Verification items for the finished model (mm, model axes). Round coordinates to 2 decimals unless told otherwise and drop trailing zeros. Order: outer loops, then holes, each group sorted by start corner. A loop starts at its lowest first (then second) coordinate and runs counter-clockwise, first axis right, second up. Notation, with made-up numbers: (-25.5, -12) -> (17.5, -12) arc R22 cw to (17.5, 26) -> close; hole circle Ø11 at (18.25, 18). An arc over 180 degrees is marked (long way). Answer in a Markdown table with one row per item. Add a question column.
```python
from build123d import *

# Parameters (mm, degrees)
F0_R = 4.953


with BuildPart() as f2:
    # F2: sweep along a path in F1
    with BuildLine(Plane.YZ) as f2_path:
        Line((0, 0), (0, 152.4))
        Line((0, 152.4), (304.8, 152.4))
        Line((304.8, 152.4), (304.8, -609.6))
        Line((304.8, -609.6), (1371.6, -609.6))
        Line((1371.6, -609.6), (1371.6, -457.2))
    # F0 (on Top) → F2 (sweep)
    with BuildSketch(Plane.XY):
        Circle(F0_R)
    sweep(path=f2_path.line, transition=Transition.RIGHT)


solid = f2.part
```
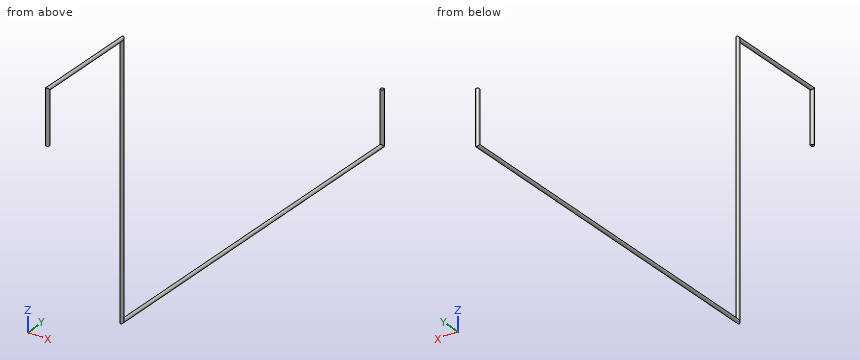
1) Depth check by flat-ended pin: P1, Ø1, axis at x = 1.5, z = -277.5, coming from the +Y side; P2, Ø2, axis at x = 2, y = 239, coming from the -Z side; P3, Ø3, axis at x = -2, y = 584, coming from the -Z side. Enter the tip coordinate at first touch or a pass-through.
2) Cross-section at D-D, the plane z = -320.5. Record the boundary of the cut face in (x, y).
3) Cross-section at A-A, the plane x = 0. Record the boundary of the cut face in (y, z).
4) Thickness scan on L1, parallel to Y at x = 1.25, z = 12.5; L2, parallel to Y at x = 0.5, z = -463; L3, parallel to Z at x = 1.5, y = 196. Record the ranges inside material, lowest first. Write a range as [from, to].
5) Cross-section at C-C, the plane y = 550.5. Record the boundary of the cut face in (x, z).
6) Cross-section at B-B, the plane z = 93. Record the boundary of the cut face in (x, y).
Results below:
| question | item | result |
|---|---|---|
| 1 | P1 | y = 309.65 |
| 1 | P2 | z = 147.55 |
| 1 | P3 | z = -614.53 |
| 2 | outline | circle Ø9.91 at (0, 304.8) |
| 3 | outline | (-4.95, 0) -> (4.95, 0) -> (4.95, 147.45) -> (299.85, 147.45) -> (299.85, -614.55) -> (1376.55, -614.55) -> (1376.55, -457.2) -> (1366.65, -457.2) -> (1366.65, -604.65) -> (309.75, -604.65) -> (309.75, 157.35) -> (-4.95, 157.35) -> close |
| 4 | L1 | [-4.79, 4.79], [300.01, 309.59] |
| 4 | L2 | [299.87, 309.73], [1366.67, 1376.53] |
| 4 | L3 | [147.68, 157.12] |
| 5 | outline | circle Ø9.91 at (0, -609.6) |
| 6 | outline | circle Ø9.91 at (0, 0); circle Ø9.91 at (0, 304.8) |
